Read the model definition and answer for the solid it produces. Units are mm, in the model's axes. Give positions to 0.01 mm unless a question says otherwise; leave off trailing zeros. Order: outer loops, then holes, each group sorted by start corner. A loop starts at its lowest first (then second) coordinate and runs counter-clockwise, first axis right, second up. Notation, with made-up numbers: (-12, -40) - (5, -40) arc R27 cw to (5, -17) - close; hole circle Ø6 at (-36.5, 6). An arc over 180 degrees is marked (long way). One line per item, written item: value. Start each with the question number.
```python
from build123d import *

# Parameters (mm, degrees)
CYLINDER2204_R     = 1
CYLINDER2204_DEPTH = 20
CYLINDER2203_R     = 1
CYLINDER2203_DEPTH = 20
BOX850_W           = 2
BOX850_H           = 7
BOX850_DEPTH       = 28
CHAMFER069_SIZE    = 1.5


with BuildPart() as obj1:
    # Cylinder2204 → Cylinder2204 (new body)
    with BuildSketch(Plane(origin=(-17, -108, 18), x_dir=(0, 0, -1), z_dir=(1, 0, 0))):
        Circle(CYLINDER2204_R)
    extrude(amount=CYLINDER2204_DEPTH)


with BuildPart() as compound986:
    # Cylinder2203 → Cylinder2203 (new body)
    with BuildSketch(Plane(origin=(-17, -108, 2), x_dir=(0, 0, -1), z_dir=(1, 0, 0))):
        Circle(CYLINDER2203_R)
    extrude(amount=CYLINDER2203_DEPTH)

    # Compound986: union obj1
    add(obj1.part)


with BuildPart() as chamfer069:
    # Box850 → Box850 (new body)
    with BuildSketch(Plane(origin=(-14.1, -111, -4), x_dir=(1, 0, 0), z_dir=(0, 0, 1))):
        with Locations((1, 3.5)):
            Rectangle(BOX850_W, BOX850_H)
    extrude(amount=BOX850_DEPTH)

    # Cut811: cut Compound986
    add(compound986.part, mode=Mode.SUBTRACT)

    # Chamfer069
    chamfer069_edges = [chamfer069.edges().sort_by_distance(p)[0] for p in [
        (-14.1, -107.5, 24),
        (-14.1, -107.5, -4),
    ]]
    chamfer(chamfer069_edges, length=CHAMFER069_SIZE)


solid = chamfer069.part
```
1) The mould has two halves that part along Z. Classify faces 1 (the flat face through (-13, -111, 10)), 2 (the flat face through (-13.3, -107.5, 23.3)), 3 (the flat face through (-13.3, -107.5, -3.3)), 4 (the cylindrical face through (-13, -109, 2)): +Z half, -Z half, draft (parallel to the pull), parting line (faces both ways), or undercut.
2) Find the intervals of material crossed by probe 1 along Y at (x, z) = (-12.85, 18); probe 2 along Z at (x, y) = (-12.45, -108.75); probe 3 along Z at (x, y) = (-12.3, -108), in increasing order. Write a range as from..to.
3) Section A-A on z = 18 is taken. Write down the section's boundary in (x, y).
4) Section B-B on y = -108 is taken. Write down the section's boundary in (x, z), plus the area to 4 significant figures.
5) Section D-D on y = -105 is taken. Write down the section's boundary in (x, z), plus the area to 4 significant figures.
6) Section C-C on x = -13.7 is taken. Write down the section's boundary in (y, z), plus the area to 3 significant figures.
Solved:
1. face 1: draft
1. face 2: +Z half
1. face 3: -Z half
1. face 4: undercut
2. probe 1: y = -111..-109, -107..-104
2. probe 2: z = -4..1.34, 2.66..17.34, 18.66..24
2. probe 3: z = -4..1, 3..17, 19..24
3. outline: (-14.1, -111) - (-12.1, -111) - (-12.1, -109) - (-14.1, -109) - close; (-14.1, -107) - (-12.1, -107) - (-12.1, -104) - (-14.1, -104) - close
4. outline: (-14.1, -2.5) - (-12.6, -4) - (-12.1, -4) - (-12.1, 1) - (-14.1, 1) - close; (-14.1, 3) - (-12.1, 3) - (-12.1, 17) - (-14.1, 17) - close; (-14.1, 19) - (-12.1, 19) - (-12.1, 24) - (-12.6, 24) - (-14.1, 22.5) - close
4. area: 45.75 mm2
5. outline: (-14.1, -2.5) - (-12.6, -4) - (-12.1, -4) - (-12.1, 24) - (-12.6, 24) - (-14.1, 22.5) - close
5. area: 53.75 mm2
6. outline: (-111, -2.9) - (-104, -2.9) - (-104, 22.9) - (-111, 22.9) - close; hole circle Ø2 at (-108, 2); hole circle Ø2 at (-108, 18)
6. area: 174 mm2
